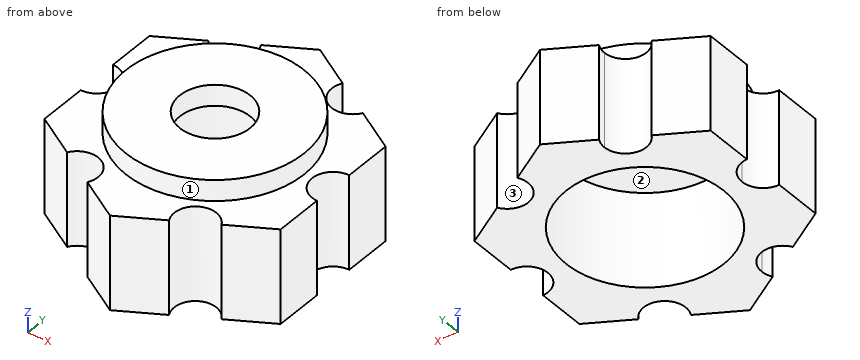
```python
from build123d import *

# Parameters (mm, degrees)
F0_R     = 8.5
F1_DEPTH = 9
F0_R_2   = 3.35
F2_DEPTH = 11
F3_R     = 7.5
F3_R_2   = 3.35
F4_DEPTH = 9


with BuildPart() as f1:
    # F0 (on Top) → F1 (new body)
    with BuildSketch(Plane.XY):
        with BuildLine():
            Line((-11.25833, -2), (-11.25833, -6.5))
            Line((-11.25833, -6.5), (-7.361216, -8.75))
            ThreePointArc((-7.361216, -8.75), (-5.111527, -7.818148), (-3.629165, -9.75))
            ThreePointArc((-3.629165, -9.75), (-3.697313, -10.267638), (-3.897114, -10.75))
            Line((-3.897114, -10.75), (0, -13))
            Line((0, -13), (3.897114, -10.75))
            ThreePointArc((3.897114, -10.75), (4.629165, -8.017949), (7.361216, -8.75))
            Line((7.361216, -8.75), (11.25833, -6.5))
            Line((11.25833, -6.5), (11.25833, -2))
            ThreePointArc((11.25833, -2), (9.25833, 0), (11.25833, 2))
            Line((11.25833, 2), (11.25833, 6.5))
            Line((11.25833, 6.5), (7.361216, 8.75))
            ThreePointArc((7.361216, 8.75), (4.629165, 8.017949), (3.897114, 10.75))
            Line((3.897114, 10.75), (0, 13))
            Line((0, 13), (-3.897114, 10.75))
            ThreePointArc((-3.897114, 10.75), (-3.697313, 10.267638), (-3.629165, 9.75))
            ThreePointArc((-3.629165, 9.75), (-5.111527, 7.818148), (-7.361216, 8.75))
            Line((-7.361216, 8.75), (-11.25833, 6.5))
            Line((-11.25833, 6.5), (-11.25833, 2))
            ThreePointArc((-11.25833, 2), (-9.844117, 1.414214), (-9.25833, 0))
            ThreePointArc((-9.25833, 0), (-9.844117, -1.414214), (-11.25833, -2))
        make_face()
        Circle(F0_R, mode=Mode.SUBTRACT)
    extrude(amount=F1_DEPTH)

    # F0 (on Top) → F2 (join)
    with BuildSketch(Plane.XY):
        Circle(F0_R)
        Circle(F0_R_2, mode=Mode.SUBTRACT)
    extrude(amount=F2_DEPTH)

    # F3 (on face) → F4 (cut)
    with BuildSketch(Plane(origin=(0, 0, 0), x_dir=(1, 0, 0), z_dir=(0, 0, -1))):
        Circle(F3_R)
        Circle(F3_R_2, mode=Mode.SUBTRACT)
    extrude(amount=-F4_DEPTH, mode=Mode.SUBTRACT)


solid = f1.part
```
CAD build for the part. Positions are in the model's coordinates, mm. Face numbers are marked on the shaded views. A direction names the side the tool comes from. Round coordinates to 2 decimals unless told otherwise and drop trailing zeros. Order: outer loops, then holes, each group sorted by start corner. A loop starts at its lowest first (then second) coordinate and runs counter-clockwise, first axis right, second up. Notation, with made-up numbers: (1.25, 73.25) - (54.25, 73.25) arc R15 cw to (54.25, 89.25) - close; hole circle Ø7 at (86, 21). An arc over 180 degrees is marked (long way). Answer in a Markdown table with one row per item. Add a question column.
(1) Band-saw the part on A-A on z = 8.25. List the corners of the cut face in (x, y), and give its area (3 significant figures).
(2) 3-axis set-ups, long thin cutter, end or side, ignore diameter. For the marked faces 1, 2 and 3: which of +Z, -Z, +X, -X, +Y, -Y reach the whole face in a straight line?
(3) Drop flat-ended pins along their axis: pin 1 Ø9 at (x, y) = (0, 0) entering from -Z; pin 2 Ø1 at (x, z) = (2, 7) entering from +Y; pin 3 Ø1.5 at (x, z) = (6, 9.5) entering from -Y. Give the stop position or say it passes through.
(4) Probe L1, parallel to Y at x = 0, z = 9.8; L2, parallel to X at y = 0, z = 3; L3, parallel to Y at x = 2.5, z = 3.75. List the from-to ranges inside material, lowest first. Write a range as [from, to].
(5) Band-saw the part on B-B on x = 7. List the corners of the cut face in (y, z).
(6) Band-saw the part on C-C on y = -5.5. List the corners of the cut face in (x, z), and give its area (3 significant figures).
Data:
| question | item | result |
|---|---|---|
| 1 | outline | (-11.26, -6.5) - (-7.36, -8.75) arc R2 cw to (-3.63, -9.75) arc R2 cw to (-3.9, -10.75) - (0, -13) - (3.9, -10.75) arc R2 cw to (7.36, -8.75) - (11.26, -6.5) - (11.26, -2) arc R2 cw to (11.26, 2) - (11.26, 6.5) - (7.36, 8.75) arc R2 cw to (3.9, 10.75) - (0, 13) - (-3.9, 10.75) arc R2 cw to (-3.63, 9.75) arc R2 cw to (-7.36, 8.75) - (-11.26, 6.5) - (-11.26, 2) arc R2 cw to (-11.26, -2) - close; hole circle Ø15 at (0, 0) |
| 1 | area | 225 mm^2 |
| 2 | face 1 | +Z |
| 2 | face 2 | -Z |
| 2 | face 3 | +Z, -Z |
| 3 | pin 1 | stops at z = 9 |
| 3 | pin 2 | stops at y = 12.13 |
| 3 | pin 3 | stops at y = -7.98 |
| 4 | L1 | y = [-8.5, -3.35], [3.35, 8.5] |
| 4 | L2 | x = [-9.26, -7.5], [7.5, 9.26] |
| 4 | L3 | y = [-11.56, -7.07], [7.07, 11.56] |
| 5 | outline | (-8.29, 0) - (-2.69, 0) - (-2.69, 9) - (2.69, 9) - (2.69, 0) - (8.29, 0) - (8.29, 9) - (4.82, 9) - (4.82, 11) - (-4.82, 11) - (-4.82, 9) - (-8.29, 9) - close |
| 6 | outline | (-11.26, 0) - (-5.1, 0) - (-5.1, 9) - (5.1, 9) - (5.1, 0) - (11.26, 0) - (11.26, 9) - (6.48, 9) - (6.48, 11) - (-6.48, 11) - (-6.48, 9) - (-11.26, 9) - close |
| 6 | area | 137 mm^2 |
